from build123d import *

# Parameters (mm, degrees)
F1_DEPTH = 25
F2_SIZE2 = 74.99999
F2_SIZE  = 17.49999


# Not quite as in the source:
# - a fillet or chamfer is up to 0.001 mm smaller than in the source, because OpenCascade refuses the exact size


with BuildPart() as f1:
    # F0 (on Front) → F1 (new body, symmetric)
    with BuildSketch(Plane.XZ):
        Polygon((25, -29.9881670944), (7.5, 45.0118329056), (-7.5, 45.0118329056), (-25, -29.9881670944), align=None)
    extrude(amount=F1_DEPTH, both=True)

    # F2 (size 17.5 and 75 in the source; OpenCascade refuses exactly that, so slightly less here)
    f2_edges = [f1.edges().sort_by_distance(p)[0] for p in [
        (0, 25, 45.011833),
        (0, -25, 45.011833),
    ]]
    f2_side = f1.faces().sort_by_distance((0, 0, 45.011833))[0]
    chamfer(f2_edges, length=F2_SIZE, length2=F2_SIZE2, reference=f2_side)


solid = f1.part
Work out the finished part from the listing and answer in its coordinate system (mm). Coordinates: 2 decimals unless noted, no trailing zeros. Loops run counter-clockwise (first coordinate to the right, second up) from the corner with the lowest first, then second, coordinate; pieces in that order, holes last. Notation, with made-up numbers: (38, 75.5) -> (49, 75.5) arc R19 cw to (49, 95.5) -> close; hole circle Ø6 at (-9.5, 8.5). An arc over 180 degrees is marked (long way). Write each question's results on one line, items separated by ' | '. Start each with the question number.
1) Find section B-B on y = 0.5. Determine the outline of the cut face in (x, z), then the cut area to 3 significant figures.
2) Consider line 1 along X through (y, z) = (6, 25.5); line 2 along Y through (x, z) = (4, 39); line 3 along Y through (x, z) = (7.5, 30). Determine where each line is inside the solid, lowest interval first.
3) Find section C-C on z = -5.5. Determine the outline of the cut face in (x, y).
4) Flat-ended cylindrical pins translate along their axes: P1, Ø1.5, axis at y = -7.5, z = -5, coming from the -X side; P2, Ø5, axis at x = -17, z = 19, coming from the +Y side; P3, Ø12, axis at y = -1.5, z = 28, coming from the -X side; P4, Ø5, axis at x = 16, z = -9.5, coming from the -Y side. Find the tip coordinate at first contact, or state that the pin passes through.
Response values:
1) outline: (-25, -29.99) -> (25, -29.99) -> (7.5, 45.01) -> (-7.5, 45.01) -> close | area: 2,440 mm^2
2) line 1: x = -12.05 to 12.05 | line 2: y = -8.9 to 8.9 | line 3: y = -11 to 11
3) outline: (-19.29, -19.29) -> (19.29, -19.29) -> (19.29, 19.29) -> (-19.29, 19.29) -> close
4) P1: stops at x = -19.34 | P2: passes through | P3: stops at x = -12.87 | P4: stops at y = -20.8
